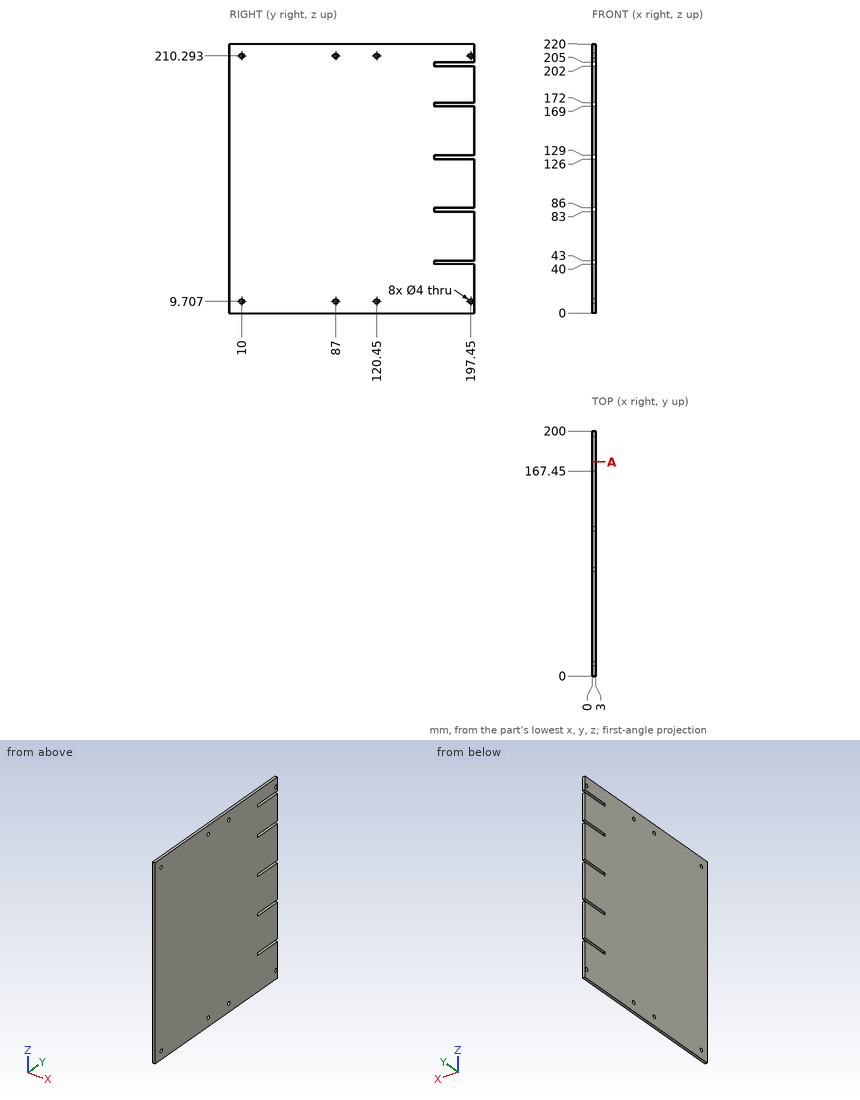
Design review of the part shown in the three views and the two pictorial views. Dimensions are in mm from the part's minimum x, y and z. Coordinates: 2 decimals unless noted, no trailing zeros. Write each loop counter-clockwise with the first axis right and the second up, starting at its lowest first coordinate (ties: lowest second). Pieces come first, ordered by that corner, then holes.
(1) Wall thickness on probe 1 along Z at (x, y) = (2.2, 10); probe 2 along Z at (x, y) = (0.95, 120); probe 3 along Z at (x, y) = (2.1, 186): over which ranges is each line inside the solid? List them lowest first.
(2) Add section A-A on y = 175. Give the boundary of the cut face in (x, z).
(3) For pin 1 Ø1.5 at (x, z) = (1, 84) entering from +Y, flat-tipped, find the tip position at first contact; note if it passes through.
Answer sheet:
1. probe 1: z = 0 to 7.71, 11.71 to 208.29, 212.29 to 220
1. probe 2: z = 0 to 7.76, 11.66 to 208.34, 212.24 to 220
1. probe 3: z = 0 to 40, 43 to 83, 86 to 126, 129 to 169, 172 to 202, 205 to 220
2. outline: (0, 0) - (3, 0) - (3, 40) - (0, 40) - close; (0, 43) - (3, 43) - (3, 83) - (0, 83) - close; (0, 86) - (3, 86) - (3, 126) - (0, 126) - close; (0, 129) - (3, 129) - (3, 169) - (0, 169) - close; (0, 172) - (3, 172) - (3, 202) - (0, 202) - close; (0, 205) - (3, 205) - (3, 220) - (0, 220) - close
3. pin 1: stops at y = 167.45
